Can you work these out from the model? Positions are in its coordinate system, mm. A direction names the side the tool comes from. Give positions to 0.01 mm unless a question says otherwise; leave off trailing zeros. Order: outer loops, then holes, each group sorted by start corner. A loop starts at its lowest first (then second) coordinate and runs counter-clockwise, first axis right, second up.
Item 1: I want a section at B-B, the plane x = -62. Write out the boundary of the cut face in (y, z), then the cut area to 3 significant figures.
Item 2: If I drill on line 1 along Z through (x, y) = (-5, -3.5); line 2 along X through (y, z) = (-6, 39); line 3 along X through (y, z) = (4, 2), over which ranges is the centre line in solid material (lowest first)?
Item 3: I'm going to push flat-ended pins straight in: pin 1 Ø15 at (x, y) = (-29.5, -1) entering from -Z; pin 2 Ø2.5 at (y, z) = (-5.3, 3.3) entering from +X; pin 3 Ø15 at (y, z) = (1, 38.5) entering from +X. Where does each tip first touch, or does it pass through?
Item 4: I want a section at D-D, the plane x = -17. Write out the boundary of the cut face in (y, z), then the cut area to 3 significant figures.
Item 5: If we mould it in two halves opening along Z, with no side actions, what happens to faces 1 (the flat face through (-78, -15, 61)), 2 (the flat face through (-77.535, 13.017, 28.574)), 3 (the cylindrical face through (-76.48, 6.28, -7.52))? For each: +Z half, -Z half, draft (parallel to the pull), parting line (faces both ways), or undercut.
Item 6: I want a section at C-C, the plane z = 50.5. Write out the boundary of the cut face in (x, y), then the cut area to 3 significant figures.
Item 7: Which directions (+Z, -Z, +X, -X, +Y, -Y) give clear straight access to the entire face, cutting with the end or side of a thin tool? Please do faces 4 (the flat face through (-65, 4, 49)), 5 (the flat face through (-34, 0, 59)), 6 (the cylindrical face through (-79, 0.2, 9.5)).
Item 8: I want a section at A-A, the plane y = 0. Write out the boundary of the cut face in (x, z), then the cut area to 3 significant figures.
```python
from build123d import *

# Parameters (mm, degrees)
CYLINDER067_R             = 11.5
CYLINDER067_DEPTH         = 23
CYLINDER066_R             = 5
CYLINDER066_DEPTH         = 23
CYLINDER068_R             = 1
CYLINDER068_DEPTH         = 31
CYLINDER071_R             = 1
CYLINDER071_DEPTH         = 31
CYLINDER070_R             = 1
CYLINDER070_DEPTH         = 31
CYLINDER069_R             = 1
CYLINDER069_DEPTH         = 31
FUSION058_ROLL_ANGLE      = -90
FUSION059_PITCH_ANGLE     = -45
FUSION059_PLACEMENT_ANGLE = 90
BOX068_W                  = 85
BOX068_H                  = 30
BOX068_DEPTH              = 4
PAD006_DEPTH              = 5
BOX069_W                  = 27
BOX069_H                  = 8
BOX069_DEPTH              = 30
CHAMFER013_SIZE           = 25


with BuildPart() as cylinder179:
    # Cylinder067 → Cylinder067 (new body)
    with BuildSketch(Plane(origin=(-3, 71, 73), x_dir=(0, 0, 1), z_dir=(0, -1, 0))):
        Circle(CYLINDER067_R)
    extrude(amount=CYLINDER067_DEPTH)


with BuildPart() as fusion057:
    # Cylinder066 → Cylinder066 (new body)
    with BuildSketch(Plane(origin=(-3, 66, 73), x_dir=(0, 0, 1), z_dir=(0, -1, 0))):
        Circle(CYLINDER066_R)
    extrude(amount=CYLINDER066_DEPTH)

    # Fusion057: union Cylinder179
    add(cylinder179.part)


with BuildPart() as cylinder180:
    # Cylinder068 → Cylinder068 (new body)
    with BuildSketch(Plane(origin=(-7.5, -11, 132), x_dir=(1, 0, 0), z_dir=(0, 0, 1))):
        Circle(CYLINDER068_R)
    extrude(amount=CYLINDER068_DEPTH)


with BuildPart() as cylinder183:
    # Cylinder071 → Cylinder071 (new body)
    with BuildSketch(Plane(origin=(0, -3.5, 132), x_dir=(1, 0, 0), z_dir=(0, 0, 1))):
        Circle(CYLINDER071_R)
    extrude(amount=CYLINDER071_DEPTH)


with BuildPart() as cylinder182:
    # Cylinder070 → Cylinder070 (new body)
    with BuildSketch(Plane(origin=(7.5, -11, 132), x_dir=(1, 0, 0), z_dir=(0, 0, 1))):
        Circle(CYLINDER070_R)
    extrude(amount=CYLINDER070_DEPTH)


with BuildPart() as fusion059:
    # Cylinder069 → Cylinder069 (new body)
    with BuildSketch(Plane(origin=(0, -18.5, 132), x_dir=(1, 0, 0), z_dir=(0, 0, 1))):
        Circle(CYLINDER069_R)
    extrude(amount=CYLINDER069_DEPTH)

    # Fusion058: union Cylinder180, Cylinder183, Cylinder182
    add(cylinder180.part)
    add(cylinder183.part)
    add(cylinder182.part)


with BuildPart() as fusion059_1:
    # Fusion058 roll: moved
    add(fusion059.part.rotate(Axis((0, 0, 0), (1, 0, 0)), FUSION058_ROLL_ANGLE))


with BuildPart() as fusion059_2:
    # Fusion058 placement: moved
    add(fusion059_1.part.moved(Location((-3, -97.5, 62))))

    # Fusion059: union Fusion057
    add(fusion057.part)


with BuildPart() as fusion059_3:
    # Fusion059 pitch: moved
    add(fusion059_2.part.rotate(Axis((0, 0, 0), (0, 1, 0)), FUSION059_PITCH_ANGLE))


with BuildPart() as fusion059_4:
    # Fusion059 placement: moved
    add(fusion059_3.part.moved(Location((-30, 53.740115, -51.497475))).rotate(Axis((-30, 53.740115, -51.497475), (0, 0, 1)), FUSION059_PLACEMENT_ANGLE))


with BuildPart() as cube071:
    # Box068 → Box068 (new body)
    with BuildSketch(Plane(origin=(-76, -15, 59), x_dir=(1, 0, 0), z_dir=(0, 0, 1))):
        with Locations((42.5, 15)):
            Rectangle(BOX068_W, BOX068_H)
    extrude(amount=BOX068_DEPTH)


with BuildPart() as fusion061:
    # Sketch008 → Pad006 (new body)
    with BuildSketch(Plane(origin=(-80, 0, 0), x_dir=(0, -1, 0), z_dir=(-1, 0, 0))):
        with BuildLine():
            ThreePointArc((-10.976703, -2.715538), (0, -13), (10.976703, -2.715538))
            Line((15.000001, 59), (10.976703, -2.715538))
            Line((15.000001, 63), (15.000001, 59))
            Line((-14.999999, 63), (15.000001, 63))
            Line((-14.999999, 63), (-14.999999, 59))
            Line((-14.999999, 59), (-10.976703, -2.715538))
        make_face()
    extrude(amount=-PAD006_DEPTH)

    # Fusion061: union Cube071
    add(cube071.part)


with BuildPart() as cut095:
    # Box069 → Box069 (new body)
    with BuildSketch(Plane(origin=(-76, -4, 33), x_dir=(1, 0, 0), z_dir=(0, 0, 1))):
        with Locations((13.5, 4)):
            Rectangle(BOX069_W, BOX069_H)
    extrude(amount=BOX069_DEPTH)

    # Chamfer013
    chamfer013_edges = [cut095.edges().sort_by_distance(p)[0] for p in [
        (-49, 0, 33),
    ]]
    chamfer(chamfer013_edges, length=CHAMFER013_SIZE)

    # Fusion062: union Fusion061
    add(fusion061.part)

    # Cut095: cut Fusion059
    add(fusion059_4.part, mode=Mode.SUBTRACT)


solid = cut095.part
```
Results list:
1. outline: (-15, 59) - (-4, 59) - (-4, 45) - (4, 45) - (4, 59) - (15, 59) - (15, 63) - (-15, 63) - close
1. area: 232 mm2
2. line 1: z = 59 to 63
2. line 2: x = -80 to -75
2. line 3: x = -78 to -75
3. pin 1: stops at z = 59
3. pin 2: stops at x = -75
3. pin 3: stops at x = -61
4. outline: (-15, 59) - (15, 59) - (15, 63) - (-15, 63) - close
4. area: 120 mm2
5. face 1: draft
5. face 2: -Z half
5. face 3: undercut
6. outline: (-80, -14.45) - (-75, -14.45) - (-75, -4) - (-56.5, -4) - (-56.5, 4) - (-75, 4) - (-75, 14.45) - (-80, 14.45) - close
6. area: 292 mm2
7. face 4: -Z, +X, +Y
7. face 5: -Z, +X
7. face 6: -Z, -X
8. outline: (-80, 9.5) - (-78, 9.5) - (-78, 3) - (-75, 3) - (-75, 33) - (-74, 33) - (-49, 58) - (-49, 59) - (9, 59) - (9, 63) - (-80, 63) - close; (-78, -13) - (-75, -13) - (-75, -7) - (-78, -7) - close
8. area: 1,000 mm2
